Source: CAD feature listing. Evaluate the final solid. Frame: model axes, mm. A direction names the side the tool comes from. Coordinates: 2 decimals unless noted, no trailing zeros. Order: outer loops, then holes, each group sorted by start corner. A loop starts at its lowest first (then second) coordinate and runs counter-clockwise, first axis right, second up. Notation, with made-up numbers: (5.25, 9) - (48.25, 9) arc R6 ccw to (48.25, 18) - close; hole circle Ø4 at (66.25, 17). An arc over 180 degrees is marked (long way). One line per question, with ' | ' between items.
from build123d import *

# Parameters (mm, degrees)
CUT_EXTRUDE1_REACH = 78.278
SKETCH2_R          = 22.225
SKETCH2_R_2        = 21.59


with BuildPart() as part:
    # Sketch1 → Revolve1 (revolve)
    with BuildSketch(Plane.XY, mode=Mode.PRIVATE) as revolve1_sk:
        Polygon((22.86, 0), (22.86, -64.42075), (0, -64.42075), (0, -62.89675), (20.955, -62.89675), (20.955, 4.66725), (22.225, 4.66725), (22.225, 2.286), (21.59, 2.286), (21.59, 0), (22.225, 0), align=None)
    revolve(revolve1_sk.sketch.rotate(Axis((0, 33.267670174, 0), (0, -1, 0)), 90), axis=Axis((0, 33.267670174, 0), (0, -1, 0)))

    # Sketch2 → Cut-Extrude1 (cut, up to next)
    with BuildSketch(Plane(origin=(0, 4.66725, 0), x_dir=(1, 0, 0), z_dir=(0, 1, 0)), mode=Mode.PRIVATE) as cut_extrude1_sk1:
        Circle(SKETCH2_R)
        with Locations(Location((0, 0, 0), (0, 0, 270))):
            Circle(SKETCH2_R_2, mode=Mode.SUBTRACT)
    cut_extrude1_tool1 = extrude(cut_extrude1_sk1.sketch, amount=-CUT_EXTRUDE1_REACH, mode=Mode.PRIVATE) & part.part
    add(cut_extrude1_tool1.solids().sort_by_distance((-21.596382, 4.66725, 0))[0], mode=Mode.SUBTRACT)


solid = part.part
(1) Pin query (flat end, axial travel): P1, Ø13.5, axis at x = -8, z = -8, coming from the +Y side; P2, Ø5, axis at x = 18, y = -40.5, coming from the -Z side; P3, Ø2, axis at y = -49.5, z = 9.5, coming from the -X side. Return the tip coordinate at first contact, or that it passes through.
Taken from the geometry:
P1: stops at y = -62.9 | P2: stops at z = -16.8 | P3: stops at x = -21.22
(2) Set-up query: faces 5 (the flat face through (0, -64.421, 0)), 6 (the flat face through (-14, 0, 17)). Return all of +Z, -Z, +X, -X, +Y, -Y with unobstructed straight access to the full face (end or side cutting, diameter ignored); none if empty.
Taken from the geometry:
face 5: +Z, -Z, +X, -X, -Y | face 6: +Y
(3) Cut plane A-A (x = 0). Return the cut outline in (y, z) (3 decimals).
Taken from the geometry:
outline: (-64.421, -22.86) - (0, -22.86) - (0, -21.59) - (4.667, -21.59) - (4.667, -20.955) - (-62.897, -20.955) - (-62.897, 20.955) - (4.667, 20.955) - (4.667, 21.59) - (0, 21.59) - (0, 22.86) - (-64.421, 22.86) - close
(4) Cut plane C-C (y = -23). Return the cut outline in (x, z) (3 decimals).
Taken from the geometry:
outline: circle Ø45.72 at (0, 0); hole circle Ø41.91 at (0, 0)
(5) Pull-direction query (Z, two-part tool) for faces 1 (the flat face through (0, -62.897, 0)), 2 (the flat face through (-3, 4.667, 21)), 3 (the cylindrical face through (-14.592, 2.301, -15.913)), 4 (the cylindrical face through (-20.777, -28.642, -2.728)); classes: pulls with the +Z half, pulls with the -Z half, needs draft (parallel to the pull), parting line crosses it, or undercut.
Taken from the geometry:
face 1: undercut | face 2: needs draft | face 3: parting line crosses it | face 4: undercut
(6) Material intervals for L1, parallel to X at y = -37, z = 0 (3 decimals); L2, parallel to Z at x = 19, y = -52; L3, parallel to Y at x = 13, z = -7.5, sorted ascending. Write a range as from..to.
Taken from the geometry:
L1: x = -22.86..-20.955, 20.955..22.86 | L2: z = -12.71..-8.84, 8.84..12.71 | L3: y = -64.42..-62.9
(7) Cut plane B-B (z = 0). Return the cut outline in (x, y) (3 decimals), and give its area (3 significant figures).
Taken from the geometry:
outline: (-22.86, -64.421) - (22.86, -64.421) - (22.86, 0) - (21.59, 0) - (21.59, 4.667) - (20.955, 4.667) - (20.955, -62.897) - (-20.955, -62.897) - (-20.955, 4.667) - (-21.59, 4.667) - (-21.59, 0) - (-22.86, 0) - close | area: 315 mm²
